Read the model definition and answer for the solid it produces. Units are mm, in the model's axes. Face numbers are marked on the shaded views. A direction names the side the tool comes from. Coordinates: 2 decimals unless noted, no trailing zeros. Write each loop counter-clockwise with the first axis right and the second up, starting at its lowest first coordinate (ties: lowest second). Pieces come first, ordered by that corner, then holes.
1) Which of the six approach directions +Z, -Z, +X, -X, +Y, -Y give full straight-line access (tool end or side, diameter ignored) to the marked faces 4, 5, 6, 7 and 8?
2) The part is cut by section B-B (x = -5). Determine the outline of the cut face in (y, z), then the cut area to 3 significant figures.
3) The part is cut by section A-A (y = 7.75). Determine the outline of the cut face in (x, z).
4) Determine the mould class of the marked faces 1, 2 and 3 for opening direction Z: +Z half, -Z half, draft (parallel to the pull), parting line (faces both ways), or undercut.
5) Each of these flat-tipped pins is pushed along its axis until it touches: pin 1 Ø1.8 at (y, z) = (7.5, -8.5) entering from +X; pin 2 Ø1.5 at (x, y) = (-4.5, 1.5) entering from -Z; pin 3 Ø4 at (x, y) = (-1.5, 10.5) entering from -Z. Where does it stop, or does it pass through?
6) The part is cut by section D-D (z = 4.75). Determine the outline of the cut face in (x, y), then the cut area to 3 significant figures.
7) The part is cut by section C-C (y = 1.25). Determine the outline of the cut face in (x, z).
8) Find the intervals of material crossed by line 1 (Y direction, x = -4.5, z = -8); line 2 (Z direction, x = -7.5, y = 9); line 3 (Y direction, x = -1, z = 4.5), in increasing order.
Autodesk Inventor part; units mm, degrees
ref_plane "YZ Plane" through (0, 0, 0) normal (1, 0, 0) x (0, 1, 0)
ref_plane "XZ Plane" through (0, 0, 0) normal (0, 1, 0) x (-1, 0, 0)
ref_plane "XY Plane" through (0, 0, 0) normal (0, 0, 1) x (1, 0, 0)
sketch "Sketch2" plane through (0, 0, 0) normal (0, 1, 0) x (-1, 0, 0)
  line L0 (0, 0) -> (7.7547, -7.7547) construction
  line L1 (0, 0) -> (0, -11.6637) construction
  line L2 (-25.4458, 33.931) -> (0, 8.4853) construction
  line L3 (0, 0) -> (8, -8)
  line L4 (8, -11.5355) -> (8, -11.5355)
  line L5 (8, -8) -> (8, -11.5355)
  line L6 (0, 0) -> (0, -3.5355)
  line L7 (0, 8.4853) -> (0.2453, 8.24)
  line L8 (0.2453, 11.7755) -> (8, 4.0208)
  line L9 (8, 4.0208) -> (8, 0.4853)
  line L10 (0.2453, 8.24) -> (8, 0.4853)
  line L11 (8, -11.5355) -> (0, -3.5355)
  line L12 (0, 8.4853) -> (8, 0.4853) construction
  line L13 (0.2453, 8.24) -> (0.2453, 11.7755)
  dimension "d0" = 45
  dimension "d1" = 6
  dimension "d2" = 2.5
  dimension "d4" = 8
extrude "Extrusion1" add sketch "Sketch2" along normal blind 12
sketch "Sketch3" plane through (0, 0, 0) normal (0, -1, 0) x (1, 0, 0)
  line L0 (-8, 4.0208) -> (-0.2453, 11.7755)
  line L1 (-8, -11.5355) -> (0, -3.5355)
  line L2 (-8, -8) -> (-8, -11.5355)
  line L3 (0, 26.3321) -> (0, -17.8468)
  line L4 (-8, 0.4853) -> (-8, 4.0208)
  line L5 (-0.2453, 11.7755) -> (0, -3.5355)
  line L6 (-8, -11.5355) -> (-8, 4.0208)
  line L7 (-8, 4.0208) -> (-0.2453, 11.7755)
  line L8 (0, -3.5355) -> (-8, -11.5355)
  point P0 (0, 0)
  point P1 (-15, -6.5147)
extrude "Extrusion2" add sketch "Sketch3" along normal blind 2.5
sketch "Sketch4" plane through (0, 0, 0) normal (0, 0, 1) x (1, 0, 0)
  line L0 (-8, 12) -> (-0.2453, 12)
  line L1 (-2.1227, 10) -> (-6.1227, 10)
  line L2 (-6.1227, 10) -> (-6.1227, 6)
  line L3 (-6.1227, 6) -> (-2.1227, 6)
  line L4 (-2.1227, 6) -> (-2.1227, 10)
  line L5 (-4.1227, 12) -> (-4.1227, 0)
  line L6 (0, 0) -> (-8, 0)
  point P0 (-4.1227, 10)
  dimension "d9" = 4
  dimension "d10" = 4
  dimension "d13" = 6
extrude "Extrusion3" cut sketch "Sketch4" along normal through all both and the other way through all
properties part number "gimbal_stick_fixation"
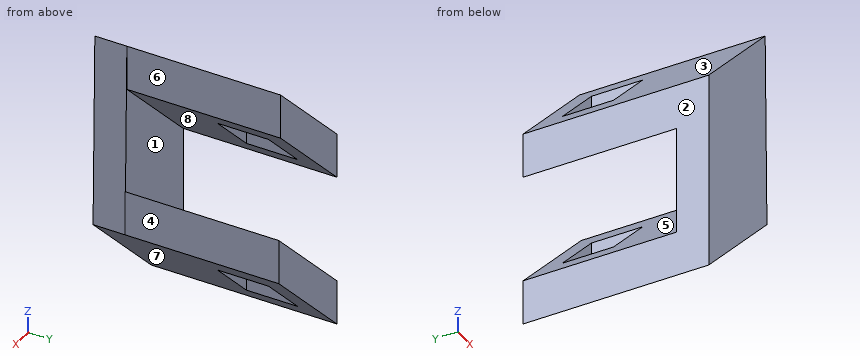
Reported:
1. face 4: +Z, -Z, +X, +Y, -Y
1. face 5: -X, +Y
1. face 6: +Z, +X, +Y
1. face 7: -Z, +X, +Y, -Y
1. face 8: +X, +Y
2. outline: (-2.5, -8.54) - (6, -8.54) - (6, -5) - (0, -5) - (0, 3.49) - (6, 3.49) - (6, 7.02) - (-2.5, 7.02) - close; (10, -8.54) - (12, -8.54) - (12, -5) - (10, -5) - close; (10, 3.49) - (12, 3.49) - (12, 7.02) - (10, 7.02) - close
2. area: 95.5 mm2
3. outline: (-8, -11.54) - (-6.12, -9.66) - (-6.12, -6.12) - (-8, -8) - close; (-8, 0.49) - (-6.12, 2.36) - (-6.12, 5.9) - (-8, 4.02) - close; (-2.12, -5.66) - (0, -3.54) - (0, 0) - (-2.12, -2.12) - close; (-2.12, 6.36) - (-0.25, 8.24) - (-0.25, 11.78) - (-2.12, 9.9) - close
4. face 1: undercut
4. face 2: draft
4. face 3: +Z half
5. pin 1: stops at x = -6.12
5. pin 2: stops at z = -8.79
5. pin 3: stops at z = -7.04
6. outline: (-7.27, -2.5) - (-0.13, -2.5) - (-0.13, 0) - (-3.74, 0) - (-3.74, 6) - (-6.12, 6) - (-6.12, 10) - (-3.74, 10) - (-3.74, 12) - (-7.27, 12) - close
6. area: 50.7 mm2
7. outline: (-8, -11.54) - (0, -3.54) - (0, 0) - (-8, -8) - close; (-8, 0.49) - (-0.25, 8.24) - (-0.25, 11.78) - (-8, 4.02) - close
8. line 1: y = -2.5 to 6, 10 to 12
8. line 2: z = -11.04 to -7.5, 0.99 to 4.52
8. line 3: y = -2.5 to 0
